Check sheet for the modelled part. Datum: model origin and axes. Units: mm. A direction names the side the tool comes from. Give positions to 0.01 mm unless a question says otherwise; leave off trailing zeros. Order: outer loops, then holes, each group sorted by start corner. A loop starts at its lowest first (then second) coordinate and runs counter-clockwise, first axis right, second up. Notation, with made-up numbers: M 73.25,39 L 79.25,39 A25 ccw 79.25,66 Z; hole C 18.25,0 d8. An arc over 180 degrees is marked long. Return JSON: item names as keys, results as strings. Group by question number.
from build123d import *

# Parameters (mm, degrees)
CROQUIS1_R                                          = 34.5
SALIENTE_EXTRUIR1_DEPTH                             = 5
CROQUIS2_R                                          = 24.5
SALIENTE_EXTRUIR2_DEPTH                             = 15
CROQUIS3_R                                          = 6.85
SALIENTE_EXTRUIR3_DEPTH                             = 30
CROQUIS4_R                                          = 2
CORTAR_EXTRUIR1_DEPTH                               = 10
MATRIZC1_COUNT                                      = 6
CORTAR_EXTRUIR2_START                               = -30
CORTAR_EXTRUIR2_DEPTH                               = 30
CUT_EXTRUDE1_START                                  = -40
CUT_EXTRUDE1_DEPTH                                  = 40
CBORE_FOR_M6_HEX_SOCKET_HEAD_CAP_SCREW1_D           = 6.6
CBORE_FOR_M6_HEX_SOCKET_HEAD_CAP_SCREW1_CBORE_D     = 11
CBORE_FOR_M6_HEX_SOCKET_HEAD_CAP_SCREW1_CBORE_DEPTH = 6.4


with BuildPart() as part:
    # Croquis1 → Saliente-Extruir1 (new body)
    with BuildSketch(Plane(origin=(0, 0, 0), x_dir=(1, 0, 0), z_dir=(0, 1, 0))):
        with Locations(Location((0, 0, 0), (0, 0, 270))):
            Circle(CROQUIS1_R)
    extrude(amount=SALIENTE_EXTRUIR1_DEPTH)

    # Croquis2 → Saliente-Extruir2 (add)
    with BuildSketch(Plane.XZ):
        with Locations(Location((0, 0, 0), (0, 0, 270))):
            Circle(CROQUIS2_R)
    extrude(amount=SALIENTE_EXTRUIR2_DEPTH)

    # Croquis3 → Saliente-Extruir3 (add)
    with BuildSketch(Plane.XZ.offset(15)):
        with Locations(Location((0, 0, 0), (0, 0, 270))):
            Circle(CROQUIS3_R)
    extrude(amount=SALIENTE_EXTRUIR3_DEPTH)

    # Croquis4 → Cortar-Extruir1 (cut)
    with BuildSketch(Plane(origin=(0, 5, 0), x_dir=(1, 0, 0), z_dir=(0, 1, 0))):
        with Locations(Location((0, 16, 0), (0, 0, 270))):
            Circle(CROQUIS4_R)
    cortar_extruir1 = extrude(amount=-CORTAR_EXTRUIR1_DEPTH, mode=Mode.SUBTRACT)

    # MatrizC1: Cortar-Extruir1 ×6 about axis
    matrizc1_axis = Axis((0, 0, 0), (0, 1, 0))
    for i in range(1, MATRIZC1_COUNT):
        add(cortar_extruir1.rotate(matrizc1_axis, i * 360 / MATRIZC1_COUNT), mode=Mode.SUBTRACT)

    # Croquis7 → Cortar-Extruir2 (cut)
    with BuildSketch(Plane.XZ.offset(45).offset(CORTAR_EXTRUIR2_START)):
        with BuildLine():
            Line((-6.37749951, 2.5), (-3.47749951, 2.5))
            Line((-3.47749951, 2.5), (-3.47749951, -2.5))
            Line((-3.47749951, -2.5), (-6.37749951, -2.5))
            ThreePointArc((-6.37749951, -2.5), (-6.85, 0), (-6.37749951, 2.5))
        make_face()
    extrude(amount=CORTAR_EXTRUIR2_DEPTH, mode=Mode.SUBTRACT)

    # Sketch1 → Cut-Extrude1 (cut)
    with BuildSketch(Plane.XZ.offset(45).offset(CUT_EXTRUDE1_START)):
        with BuildLine():
            Line((-6.37749951, -2.5), (-9.35, -2.5))
            Line((-9.35, -2.5), (-9.35, 2.5))
            Line((-9.35, 2.5), (-6.37749951, 2.5))
            ThreePointArc((-6.37749951, 2.5), (6.85, 0), (-6.37749951, -2.5))
        make_face()
    extrude(amount=CUT_EXTRUDE1_DEPTH, mode=Mode.SUBTRACT)

    # CBORE for M6 Hex Socket Head Cap Screw1 (through all)
    with Locations(Plane(origin=(0, 5, 0), x_dir=(1, 0, 0), z_dir=(0, 1, 0))):
        with Locations((0, 0)):
            CounterBoreHole(CBORE_FOR_M6_HEX_SOCKET_HEAD_CAP_SCREW1_D / 2, CBORE_FOR_M6_HEX_SOCKET_HEAD_CAP_SCREW1_CBORE_D / 2, CBORE_FOR_M6_HEX_SOCKET_HEAD_CAP_SCREW1_CBORE_DEPTH)


solid = part.part
1) Release check for a two-part mould opening along X. For faces 4 (the face through (-5, -15, -5)), 5 (the face through (7.36, -7.4, -23.37)), 6 (the face through (-3, -5, 2)) record: released by +X, released by -X, zero draft, split by the parting line, or undercut.
2) Sectioned sample at A-A on x = 0. Record the boundary of the cut face in (y, z), then the cut area to 3 significant figures.
3) Sectioned sample at D-D on y = 3.5. Record the boundary of the cut face in (x, z), then the cut area to 3 significant figures.
4) Depth check by flat-ended pin: P1, Ø3, axis at y = -2, z = 8, coming from the -X side; P2, Ø5.5, axis at x = 0, z = 0, coming from the +Y side; P3, Ø1.2, axis at x = 0.5, z = -16.5, coming from the +Y side; P4, Ø0.9, axis at x = -7.5, y = -10, coming from the -Z side. Enter the tip coordinate at first touch or a pass-through.
5) Sectioned sample at B-B on y = -9.5. Record the boundary of the cut face in (x, z).
6) Sectioned sample at C-C on z = 16. Record the boundary of the cut face in (x, y), then the cut area to 3 significant figures.
7) Material ranges on line 1 along X through (y, z) = (1.5, 8); line 2 along X through (y, z) = (-2.25, -8); line 3 along Y through (x, z) = (19, -19.5), recorded low to high.
8) Tool access check on faces 1 (the face through (8.1, 0, -23.5)), 2 (the face through (-15.84, 0.07, -7.74)), 3 (the face through (0, 5, 7)). Record the directions out of +Z, -Z, +X, -X, +Y, -Y that give a thin tool (end or side, any length) a straight path to the whole face; none if there is none.
Reply:
{
 "1": {"face 4": "zero draft", "face 5": "split by the parting line", "face 6": "undercut"},
 "2": {"outline": "M -15,-24.5 L 0,-24.5 L 0,-34.5 L 5,-34.5 L 5,-18 L -5,-18 L -5,-14 L 5,-14 L 5,-5.5 L -1.4,-5.5 L -1.4,-3.3 L -5,-3.3 L -5,-6.85 L -15,-6.85 Z; M -15,6.85 L -5,6.85 L -5,3.3 L -1.4,3.3 L -1.4,5.5 L 5,5.5 L 5,14 L -5,14 L -5,18 L 5,18 L 5,34.5 L 0,34.5 L 0,24.5 L -15,24.5 Z", "area": "769 mm^2"},
 "3": {"outline": "C 0,0 d69; hole C -13.86,-8 d4; hole C -13.86,8 d4; hole C 0,0 d11; hole C 0,-16 d4; hole C 0,16 d4; hole C 13.86,-8 d4; hole C 13.86,8 d4", "area": "3,570 mm^2"},
 "4": {"P1": "x = -23.62", "P2": "through", "P3": "y = -5", "P4": "z = -23.46"},
 "5": {"outline": "C 0,0 d49; hole M -9.35,-2.5 L -6.38,-2.5 A6.85 ccw long -6.38,2.5 L -9.35,2.5 Z"},
 "6": {"outline": "M -30.57,0 L -18.55,0 L -18.55,-15 L 18.55,-15 L 18.55,0 L 30.57,0 L 30.57,5 L 2,5 L 2,-5 L -2,-5 L -2,5 L -30.57,5 Z", "area": "822 mm^2"},
 "7": {"line 1": "-33.56 to -15.86, -11.86 to 11.86, 15.86 to 33.56", "line 2": "-23.16 to -15.86, -11.86 to 11.86, 15.86 to 23.16", "line 3": "0 to 5"},
 "8": {"face 1": "-Y", "face 2": "+Y", "face 3": "+Z, -Z, +X, -X, +Y"}
}
